Model file for the job. Use its own axes, mm. Face numbers are marked on the shaded views. A direction names the side the tool comes from. Coordinates: 2 decimals unless noted, no trailing zeros. Write each loop counter-clockwise with the first axis right and the second up, starting at its lowest first coordinate (ties: lowest second). Pieces come first, ordered by that corner, then holes. Notation, with made-up numbers: M -30.5,-7 L 14.5,-7 A25 cw 14.5,7 Z; hole C 31.25,83.5 d6. An arc over 180 degrees is marked long. Answer in a Markdown table with one row per item. Add a question column.
```python
from build123d import *

# Parameters (mm, degrees)
SKETCH_R        = 9.25
PAD_DEPTH       = 25
SKETCH001_R     = 1.75
POCKET_DEPTH    = 22.501
POCKET001_DEPTH = 3
CHAMFER_SIZE2   = 12
CHAMFER_SIZE    = 3
FILLET_R        = 3
FILLET001_R     = 3


with BuildPart() as part:
    # Sketch → Pad (new body)
    with BuildSketch(Plane.XY):
        with BuildLine():
            ThreePointArc((15, 0), (3.882286, 14.488887), (-12.990381, 7.5))
            Line((-12.990381, 7.5), (-26.990381, 7.5))
            Line((-26.990381, 7.5), (-26.990381, 2.5))
            Line((-26.990381, 2.5), (-14.990381, 2.5))
            Line((-14.990381, 2.5), (-14.990381, -2.5))
            Line((-26.990381, -2.5), (-14.990381, -2.5))
            Line((-26.990381, -7.5), (-26.990381, -2.5))
            Line((-12.990381, -7.5), (-26.990381, -7.5))
            ThreePointArc((-12.990381, -7.5), (3.882286, -14.488887), (15, 0))
        make_face()
        Circle(SKETCH_R, mode=Mode.SUBTRACT)
    extrude(amount=PAD_DEPTH)

    # Sketch001 (on Face8 of Pad) → Pocket (cut, through all)
    with BuildSketch(Plane.XZ.offset(7.5)):
        with Locations((-20, 6)):
            Circle(SKETCH001_R)
        with Locations((-20, 18)):
            Circle(SKETCH001_R)
    extrude(amount=-POCKET_DEPTH, mode=Mode.SUBTRACT)

    # Sketch002 (on Face3 of Pocket) → Pocket001 (cut)
    with BuildSketch(Plane(origin=(0, 7.5, 0), x_dir=(-1, 0, 0), z_dir=(0, 1, 0))):
        Polygon((20, 2.75), (22.814583, 4.375), (22.814583, 7.625), (20, 9.25), (17.185417, 7.625), (17.185417, 4.375), align=None)
        Polygon((20, 14.75), (22.814583, 16.375), (22.814583, 19.625), (20, 21.25), (17.185417, 19.625), (17.185417, 16.375), align=None)
    extrude(amount=-POCKET001_DEPTH, mode=Mode.SUBTRACT)

    # Chamfer
    chamfer_edges = [part.edges().sort_by_distance(p)[0] for p in [
        (-26.990381, 5, 0),
        (-26.990381, -5, 0),
    ]]
    chamfer_side = part.faces().sort_by_distance((3.748719, 13.990411, 0))[0]
    chamfer(chamfer_edges, length=CHAMFER_SIZE, length2=CHAMFER_SIZE2, reference=chamfer_side)

    # Fillet
    fillet_edges = [part.edges().sort_by_distance(p)[0] for p in [
        (-23.990381, 5, 0),
        (-23.990381, -5, 0),
    ]]
    fillet(fillet_edges, radius=FILLET_R)

    # Fillet001
    fillet001_edges = [part.edges().sort_by_distance(p)[0] for p in [
        (3.882286, -14.488887, 0),
        (3.882286, 14.488887, 0),
    ]]
    fillet(fillet001_edges, radius=FILLET001_R)


solid = part.part
```
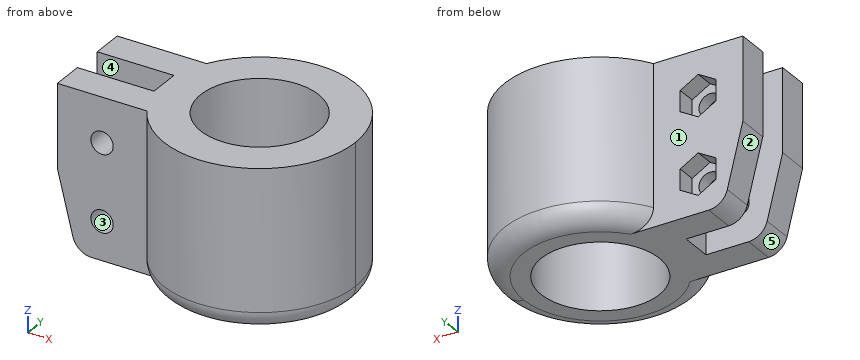
1) Slice it at B-B (z = 22.5). Give the cut face in (x, y), then the cut area to 3 significant figures.
2) Slice it at C-C (y = -4). Count the separate pieces of the cut face and the enclosed holes in it, then the cut area to 3 significant figures.
3) Flat gauge pins, fed straight in: pin 1 Ø1.7 at (x, z) = (-20, 17) entering from +Y; pin 2 Ø9 at (x, z) = (-15.5, 14.5) entering from +Y; pin 3 Ø2.5 at (y, z) = (5.5, 6.5) entering from -X; pin 4 Ø2 at (x, z) = (-20, 18) entering from +Y. Where does each tip first touch, or does it go through?
4) Which spindle directions (+Z, -Z, +X, -X, +Y, -Y) get a long thin tool onto all of the face, cutting with end or side? Do the marked faces 4 and 5. Say none if no direction does.
5) Two-plate mould, pull along X, no slides. Class the marked faces 1, 2 and 3: released by +X, released by -X, zero draft, split by the parting line, or undercut.
6) Slice it at A-A (z = 18). Give the cut face in (x, y).
7) Drill centre lines: probe 1 along Z at (x, y) = (-20, 3.6); probe 2 along Y at (x, z) = (-24.5, 12.75); probe 3 along Y at (x, z) = (-2, 5.5). Where is each one in solid material? Low to high.
8) Slice it at D-D (z = 6). Give the cut face in (x, y).
Ans:
| question | item | result |
|---|---|---|
| 1 | outline | M -26.99,-7.5 L -12.99,-7.5 A15 ccw long -12.99,7.5 L -26.99,7.5 L -26.99,2.5 L -14.99,2.5 L -14.99,-2.5 L -26.99,-2.5 Z; hole C 0,0 d18.5 |
| 1 | area | 568 mm2 |
| 2 | separate pieces | 2 |
| 2 | enclosed holes | 2 |
| 2 | area | 579 mm2 |
| 3 | pin 1 | stops at y = 4.5 |
| 3 | pin 2 | stops at y = 10.2 |
| 3 | pin 3 | stops at x = -25.93 |
| 3 | pin 4 | passes through |
| 4 | face 4 | +Z, -Z, -X |
| 4 | face 5 | -Z, -X, +Y, -Y |
| 5 | face 1 | zero draft |
| 5 | face 2 | released by -X |
| 5 | face 3 | undercut |
| 6 | outline | M -26.99,-7.5 L -21.75,-7.5 L -21.75,-2.5 L -26.99,-2.5 Z; M -26.99,2.5 L -21.75,2.5 L -21.75,4.5 L -22.81,4.5 L -22.81,7.5 L -26.99,7.5 Z; M -18.25,-7.5 L -12.99,-7.5 A15 ccw long -12.99,7.5 L -17.19,7.5 L -17.19,4.5 L -18.25,4.5 L -18.25,2.5 L -14.99,2.5 L -14.99,-2.5 L -18.25,-2.5 Z; hole C 0,0 d18.5 |
| 7 | probe 1 | z = 0 to 4.25, 7.75 to 16.25, 19.75 to 25 |
| 7 | probe 2 | y = -7.5 to -2.5, 2.5 to 7.5 |
| 7 | probe 3 | y = -14.87 to -9.03, 9.03 to 14.87 |
| 8 | outline | M -25.49,-7.5 L -21.75,-7.5 L -21.75,-2.5 L -25.49,-2.5 Z; M -25.49,2.5 L -21.75,2.5 L -21.75,4.5 L -22.81,4.5 L -22.81,7.5 L -25.49,7.5 Z; M -18.25,-7.5 L -12.99,-7.5 A15 ccw long -12.99,7.5 L -17.19,7.5 L -17.19,4.5 L -18.25,4.5 L -18.25,2.5 L -14.99,2.5 L -14.99,-2.5 L -18.25,-2.5 Z; hole C 0,0 d18.5 |
